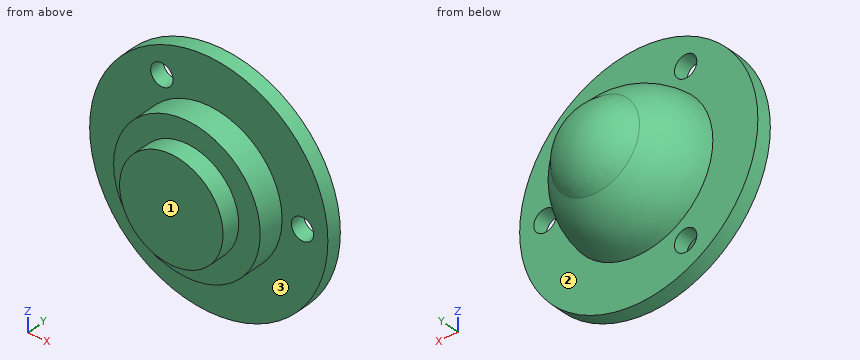
from build123d import *

# Parameters (mm, degrees)
SKETCH001_R        = 1.5
POCKET_DEPTH       = 109.668659
POLARPATTERN_COUNT = 3


with BuildPart() as part:
    # Sketch → Revolution (revolve)
    with BuildSketch(Plane.XY):
        with BuildLine():
            Line((0, 0), (0, 18.15))
            ThreePointArc((5.96381, 15), (3.373784, 17.316935), (0, 18.15))
            ThreePointArc((9.951065, 8), (8.693509, 11.919272), (5.96381, 15))
            Line((9.951065, 8), (16, 8))
            Line((16, 6), (16, 8))
            Line((9.85, 6), (16, 6))
            Line((9.85, 2.5), (9.85, 6))
            Line((6.95, 2.5), (9.85, 2.5))
            Line((6.95, 0), (6.95, 2.5))
            Line((0, 0), (6.95, 0))
        make_face()
    revolve(axis=Axis((0, 0, 0), (0, 1, 0)))

    # Sketch001 → Pocket (cut, through all)
    with BuildSketch(Plane.XZ.offset(-6)):
        with Locations((12.6, 0)):
            Circle(SKETCH001_R)
    pocket = extrude(amount=-POCKET_DEPTH, mode=Mode.SUBTRACT)

    # PolarPattern: Pocket ×3 about axis
    polarpattern_axis = Axis((0, 6, 0), (0, -1, 0))
    for i in range(1, POLARPATTERN_COUNT):
        add(pocket.rotate(polarpattern_axis, i * 360 / POLARPATTERN_COUNT), mode=Mode.SUBTRACT)


solid = part.part
Design review of the part built by this model. Coordinates are the model's own, in mm. Face numbers are marked on the shaded views. A direction names the side the tool comes from. Coordinates: 2 decimals unless noted, no trailing zeros. Order: outer loops, then holes, each group sorted by start corner. A loop starts at its lowest first (then second) coordinate and runs counter-clockwise, first axis right, second up. Notation, with made-up numbers: (-11.75, -33.5) -> (13.25, -33.5) arc R26 cw to (13.25, -18.5) -> close; hole circle Ø5 at (-30.5, -0.5). An arc over 180 degrees is marked (long way). One line per item, written item: value.
1) Machinability: for the marked faces 1, 2 and 3, which of the approach directions +Z, -Z, +X, -X, +Y, -Y give a long, thin tool a straight path to every point of the face, cutting with its end or side? Answer none if there is none.
Output values:
face 1: +Z, -Z, +X, -X, -Y
face 2: +Y
face 3: -Y
2) To check wall thickness, follow probe 1 along Z at (x, y) = (-6.3, 6.5); probe 2 along Y at (x, z) = (11, -4); probe 3 along X at (y, z) = (5, 2.5). State the ranges of each line that lie inside material, in increasing order. Write a range as [from, to].
Output values:
probe 1: z = [-14.71, -12.41], [-9.41, 9.41], [12.41, 14.71]
probe 2: y = [6, 8]
probe 3: x = [-9.53, 9.53]
3) We need section B-B, the plane y = 1.75. Give the boundary of the cut face in (x, z).
Output values:
outline: circle Ø13.9 at (0, 0)
4) We need section A-A, the plane x = 12.6. Give the boundary of the cut face in (y, z).
Output values:
outline: (6, -9.86) -> (8, -9.86) -> (8, -1.5) -> (6, -1.5) -> close; (6, 1.5) -> (8, 1.5) -> (8, 9.86) -> (6, 9.86) -> close
5) Clearance check with flat-ended pins moving along their axes: P1, Ø8, axis at y = 6, z = 3.5, coming from the +X side; P2, Ø3, axis at x = -2, y = 8.5, coming from the +Z side; P3, Ø5, axis at x = 12.6, z = 0, coming from the +Y side; P4, Ø4, axis at y = 8.5, z = -10, coming from the -X side. State where each tip first meets the part, or that it passes through.
Output values:
P1: stops at x = 16
P2: stops at z = 15.99
P3: stops at y = 8
P4: stops at x = -13.82
6) We need section C-C, the plane y = 7. Give the boundary of the cut face in (x, z), then the cut area to 3 significant figures.
Output values:
outline: circle Ø32 at (0, 0); hole circle Ø3 at (-6.3, -10.91); hole circle Ø3 at (-6.3, 10.91); hole circle Ø3 at (12.6, 0)
area: 783 mm2
